Read the model definition and answer for the solid it produces. Units are mm, in the model's axes. Face numbers are marked on the shaded views. A direction names the side the tool comes from. Round coordinates to 2 decimals unless told otherwise and drop trailing zeros. Loops run counter-clockwise (first coordinate to the right, second up) from the corner with the lowest first, then second, coordinate; pieces in that order, holes last. Notation, with made-up numbers: M -10,47.25 L 1,47.25 A21 cw 1,54.25 Z; hole C -37.5,25 d9. An arc over 180 degrees is marked long. Answer as CSV lines item,"result".
```python
from build123d import *

# Parameters (mm, degrees)
F1_DEPTH = 25.4
F2_W     = 6.35
F2_H     = 6.35
F3_DEPTH = 63.5
F4_R     = 3.175
F5_DEPTH = 63.5


with BuildPart() as f1:
    # F0 (on Front) → F1 (new body)
    with BuildSketch(Plane.XZ):
        Polygon((-4.445, 19.05), (-25.4, 19.05), (-25.4, -19.05), (25.4, -19.05), (25.4, 19.05), (4.445, 19.05), (4.445, 0), (0, 0), (-4.445, 0), align=None)
    extrude(amount=F1_DEPTH)

    # F2 (on Front) → F3 (join)
    with BuildSketch(Plane.XZ):
        with Locations((28.575, -3.175)):
            Rectangle(F2_W, F2_H)
        with Locations((28.575, 3.175)):
            Rectangle(F2_W, F2_H)
    extrude(amount=F3_DEPTH)

    # F4 (on Right) → F5 (cut, symmetric)
    with BuildSketch(Plane.YZ):
        with Locations((-57.15, 0)):
            Circle(F4_R)
    extrude(amount=F5_DEPTH, both=True, mode=Mode.SUBTRACT)


solid = f1.part
```
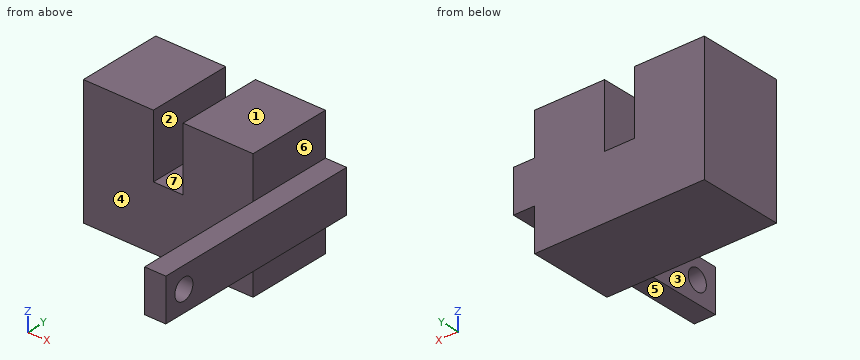
1) Find section C-C, the plane x = 27. Give the vertices of the cut face in (y, z) (3 decimals).
Evaluation:
outline,"M -63.5,-6.35 L 0,-6.35 L 0,6.35 L -63.5,6.35 Z; hole C -57.15,0 d6.35"
2) Find section B-B, the plane y = -57.15. Give the vertices of the cut face in (x, z) (3 decimals), then the cut area to 3 significant figures.
Evaluation:
outline,"M 25.4,-6.35 L 31.75,-6.35 L 31.75,-3.175 L 25.4,-3.175 Z; M 25.4,3.175 L 31.75,3.175 L 31.75,6.35 L 25.4,6.35 Z"
area,"40.3 mm^2"
3) A tool of negligible diameter and unlimited length cuts with its end or side. For the marked faces 4, 5, 6 and 7, from which of +Z, -Z, +X, -X, +Y, -Y can it reach the whole face along a straight path? Write none if from no direction.
Evaluation:
face 4,"+Z, -Z, -X, -Y"
face 5,"-Z, +X, +Y, -Y"
face 6,"+Z, +X, +Y, -Y"
face 7,"+Z, +Y, -Y"
4) Straight lines are drawn through the part: line 1 (X direction, y = -2.5, z = 10.5) (3 decimals); line 2 (X direction, y = -5.5, z = 6) (3 decimals); line 3 (Z direction, x = 30, y = -57). For each, find the intervals that lie inside material, in ascending order.
Evaluation:
line 1,"x = -25.4 to -4.445, 4.445 to 25.4"
line 2,"x = -25.4 to -4.445, 4.445 to 31.75"
line 3,"z = -6.35 to -3.17, 3.17 to 6.35"
5) Find section D-D, the plane z = 1.5. Give the vertices of the cut face in (x, y) (3 decimals), then the cut area to 3 significant figures.
Evaluation:
outline,"M -25.4,-25.4 L -4.445,-25.4 L -4.445,0 L -25.4,0 Z; M 4.445,-25.4 L 25.4,-25.4 L 25.4,-54.352 L 31.75,-54.352 L 31.75,0 L 4.445,0 Z; M 25.4,-63.5 L 31.75,-63.5 L 31.75,-59.948 L 25.4,-59.948 Z"
area,"1,430 mm^2"
6) Find section A-A, the plane z = 8. Give the vertices of the cut face in (x, y) (3 decimals).
Evaluation:
outline,"M -25.4,-25.4 L -4.445,-25.4 L -4.445,0 L -25.4,0 Z; M 4.445,-25.4 L 25.4,-25.4 L 25.4,0 L 4.445,0 Z"
7) Determine the mould class of the marked faces 1, 2 and 3 for opening direction X: released by +X, released by -X, zero draft, split by the parting line, or undercut.
Evaluation:
face 1,"zero draft"
face 2,"undercut"
face 3,"released by -X"
8) Each of these flat-tipped pins is pushed along its axis until it touches: P1, Ø21, axis at y = -11.5, z = 13, coming from the +X side; P2, Ø6, axis at y = -50, z = -3.5, coming from the -X side; P3, Ø1.5, axis at x = 23.5, y = -38, coming from the +Z side; P4, Ø6.5, axis at y = -10, z = 15.5, coming from the +X side. Where does it stop, or does it pass through?
Evaluation:
P1,"stops at x = 31.75"
P2,"stops at x = 25.4"
P3,"passes through"
P4,"stops at x = 25.4"
